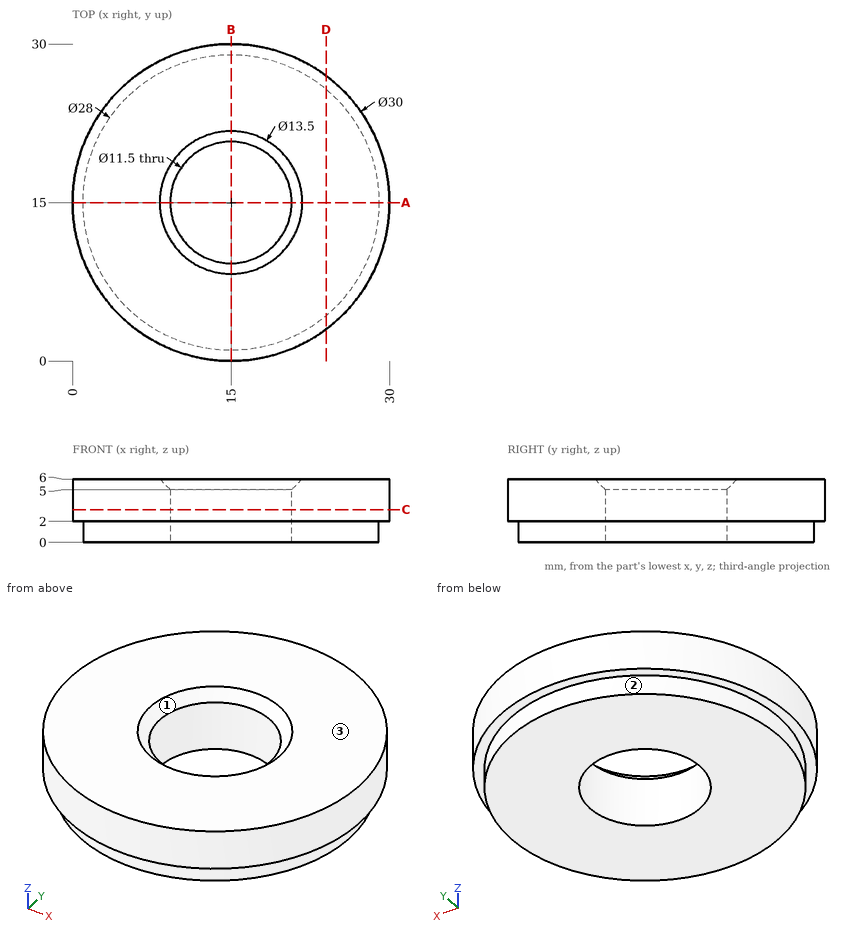
The figure shows three views and two pictorial views of one solid part (mm, origin at its lowest corner). Answer the questions. Round coordinates to 2 decimals unless told otherwise and drop trailing zeros. Loops run counter-clockwise (first coordinate to the right, second up) from the corner with the lowest first, then second, coordinate; pieces in that order, holes last. Notation, with made-up numbers: M 33.5,1.25 L 69.5,1.25 A31 ccw 69.5,31.25 Z; hole C -38,67 d11. An arc over 180 degrees is marked long. Write each question's results on one line, items separated by ' | '. Start each with the question number.
1) Find section C-C on z = 3.1. Write down the section's boundary in (x, y), plus the area to 3 significant figures.
2) Determine the mould class of the marked faces 1, 2 and 3 for opening direction Y: pulls with the +Y half, pulls with the -Y half, needs draft (parallel to the pull), parting line crosses it, or undercut.
3) Find section D-D on x = 24. Write down the section's boundary in (y, z).
4) Find section A-A on y = 15. Write down the section's boundary in (x, z), plus the area to 3 significant figures.
5) Each of these flat-tipped pins is pushed along its axis until it touches: pin 1 (1 mm diameter, centred on x = 7, z = 3, fed in from -Y); pin 2 (15 mm diameter, centred on x = 14, y = 21, fed in from -Z); pin 3 (9 mm diameter, centred on x = 15, y = 15, fed in from +Z). Where does it stop, or does it pass through?
6) Straight lines are drawn through the part: probe 1 along Y at (x, z) = (15, 3.7); probe 2 along Y at (x, z) = (15, 1.2); probe 3 along Z at (x, y) = (26.5, 24.5). For each, find the intervals that lie inside material, in ascending order.
Final values:
1) outline: C 15,15 d30; hole C 15,15 d11.5 | area: 603 mm²
2) face 1: undercut | face 2: parting line crosses it | face 3: needs draft
3) outline: M 3,2 L 4.28,2 L 4.28,0 L 25.72,0 L 25.72,2 L 27,2 L 27,6 L 3,6 Z
4) outline: M 0,2 L 1,2 L 1,0 L 9.25,0 L 9.25,5 L 8.25,6 L 0,6 Z; M 20.75,0 L 29,0 L 29,2 L 30,2 L 30,6 L 21.75,6 L 20.75,5 Z | area: 106 mm²
5) pin 1: y = 2.01 | pin 2: z = 0 | pin 3: through
6) probe 1: 0 to 9.25, 20.75 to 30 | probe 2: 1 to 9.25, 20.75 to 29 | probe 3: 2 to 6
